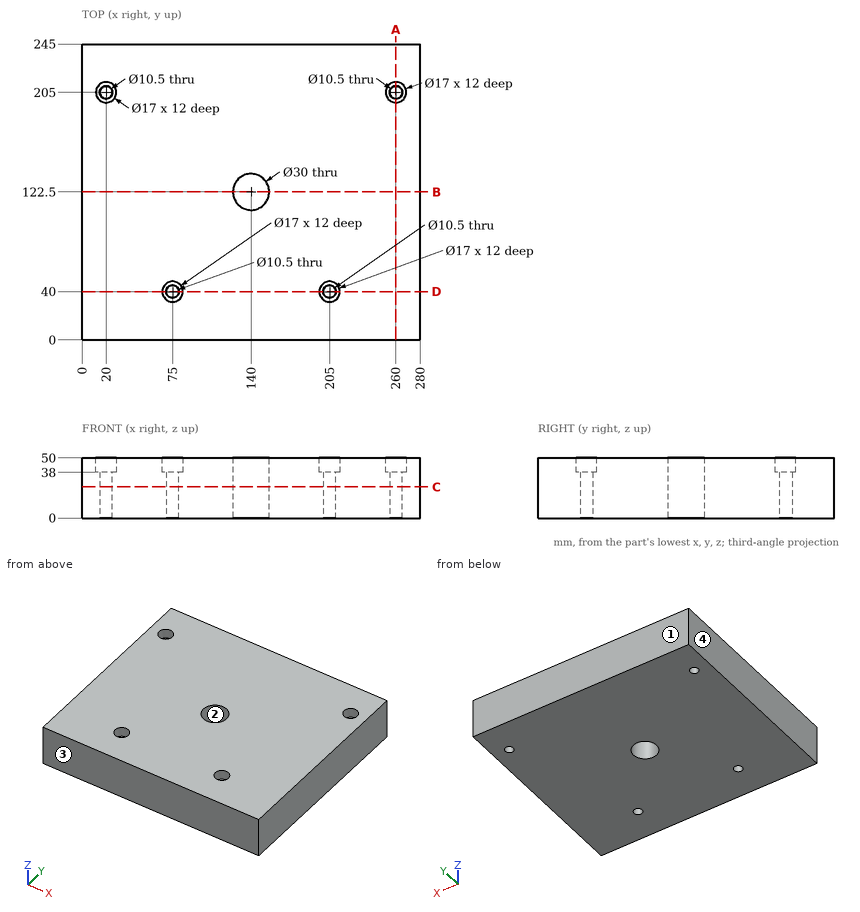
The drawing under review shows one solid part. Ordinate dimensions are in mm from its lowest x, y, z. Round coordinates to 2 decimals unless told otherwise and drop trailing zeros. Loops run counter-clockwise (first coordinate to the right, second up) from the corner with the lowest first, then second, coordinate; pieces in that order, holes last. Notation, with made-up numbers: (-26, -33) - (25, -33) arc R21 cw to (25, -18) - close; hole circle Ø5 at (84.5, 71). An arc over 180 degrees is marked (long way). Use a Markdown table: item, result. Add a question column.
Q1. Add section C-C (z = 26). State the section outline as (x, y) points.
Q2. For probe 1 along X at (y, z) = (35.5, 11); probe 2 along Y at (x, z) = (140, 24.5); probe 3 along Y at (x, z) = (20, 29), list the stretches that pass through material, from the lowest coordinate up.
Q3. Insertion check: pin 1 Ø15.5 at (x, y) = (205, 40) entering from +Z. The pin has a flat end and moves straight along its axis. Give the tip position at first contact, or say it passes through.
Q4. Add section A-A (x = 260). State the section outline as (y, z) points, plus the area to 3 significant figures.
Q5. Add section B-B (y = 122.5). State the section outline as (x, z) points.
Q6. The part is to be moulded in two halves that separate along Y. For the marked faces 1, 2, 3 and 4, say which applies: pulls with the +Y half, pulls with the -Y half, needs draft (parallel to the pull), parting line crosses it, or undercut.
Q7. Add section D-D (y = 40). State the section outline as (x, z) points, plus the area to 3 significant figures.
Worked answers:
| question | item | result |
|---|---|---|
| 1 | outline | (0, 0) - (280, 0) - (280, 245) - (0, 245) - close; hole circle Ø10.5 at (20, 205); hole circle Ø10.5 at (75, 40); hole circle Ø30 at (140, 122.5); hole circle Ø10.5 at (205, 40); hole circle Ø10.5 at (260, 205) |
| 2 | probe 1 | 0 to 72.3, 77.7 to 202.3, 207.7 to 280 |
| 2 | probe 2 | 0 to 107.5, 137.5 to 245 |
| 2 | probe 3 | 0 to 199.75, 210.25 to 245 |
| 3 | pin 1 | z = 38 |
| 4 | outline | (0, 0) - (199.75, 0) - (199.75, 38) - (196.5, 38) - (196.5, 50) - (0, 50) - close; (210.25, 0) - (245, 0) - (245, 50) - (213.5, 50) - (213.5, 38) - (210.25, 38) - close |
| 4 | area | 11,600 mm² |
| 5 | outline | (0, 0) - (125, 0) - (125, 50) - (0, 50) - close; (155, 0) - (280, 0) - (280, 50) - (155, 50) - close |
| 6 | face 1 | pulls with the +Y half |
| 6 | face 2 | undercut |
| 6 | face 3 | pulls with the -Y half |
| 6 | face 4 | needs draft |
| 7 | outline | (0, 0) - (69.75, 0) - (69.75, 38) - (66.5, 38) - (66.5, 50) - (0, 50) - close; (80.25, 0) - (199.75, 0) - (199.75, 38) - (196.5, 38) - (196.5, 50) - (83.5, 50) - (83.5, 38) - (80.25, 38) - close; (210.25, 0) - (280, 0) - (280, 50) - (213.5, 50) - (213.5, 38) - (210.25, 38) - close |
| 7 | area | 12,800 mm² |
